```python
from build123d import *

# Parameters (mm, degrees)
SKETCH007_R      = 1.625
EXTRUDE007_DEPTH = 75
SKETCH006_R      = 1.625
EXTRUDE006_DEPTH = 10
EXTRUDE004_DEPTH = 20
SKETCH005_W      = 48
SKETCH005_H      = 25
SKETCH005_R      = 1.625
EXTRUDE005_DEPTH = 5
FILLET014_R      = 1
FILLET001_R      = 1
FILLET002_R      = 0.25


with BuildPart() as extrude007:
    # Sketch007 → Extrude007 (new body)
    with BuildSketch(Plane.YZ):
        with Locations((-8.1, 14.25)):
            Circle(SKETCH007_R)
    extrude(amount=EXTRUDE007_DEPTH)


with BuildPart() as cuts:
    # Sketch006 → Extrude006 (new body)
    with BuildSketch(Plane.XY):
        with Locations((29.75, -15.85)):
            Circle(SKETCH006_R)
    extrude(amount=-EXTRUDE006_DEPTH)

    # Fusion016: union Extrude007
    add(extrude007.part)


with BuildPart() as extrude004:
    # Sketch004 → Extrude004 (new body)
    with BuildSketch(Plane.XZ):
        Polygon((25, 0), (25, -4), (59.5, -4), (59.5, 21), (55.5, 21), (55.5, 0), align=None)
    extrude(amount=EXTRUDE004_DEPTH)


with BuildPart() as fillet002:
    # Sketch005 → Extrude005 (new body)
    with BuildSketch(Plane.XZ):
        with Locations((49, 8.5)):
            Rectangle(SKETCH005_W, SKETCH005_H)
        with Locations((67, 15)):
            Circle(SKETCH005_R, mode=Mode.SUBTRACT)
        with Locations((67, 2)):
            Circle(SKETCH005_R, mode=Mode.SUBTRACT)
    extrude(amount=EXTRUDE005_DEPTH)

    # Fusion015: union Extrude004
    add(extrude004.part)

    # Cut019: cut cuts
    add(cuts.part, mode=Mode.SUBTRACT)

    # Fillet014
    fillet014_edges = [fillet002.edges().sort_by_distance(p)[0] for p in [
        (57.5, -20, 21),
        (59.5, -20, 8.5),
        (55.5, -20, 10.5),
        (25, -20, -2),
        (42.25, -20, -4),
        (40.25, -20, 0),
    ]]
    fillet(fillet014_edges, radius=FILLET014_R)

    # Fillet001
    fillet001_edges = [fillet002.edges().sort_by_distance(p)[0] for p in [
        (66.25, -5, 21),
        (66.25, -5, -4),
        (73, -5, 8.5),
    ]]
    fillet(fillet001_edges, radius=FILLET001_R)

    # Fillet002
    fillet002_edges = [fillet002.edges().sort_by_distance(p)[0] for p in [
        (59.5, -9.725, 14.25),
        (28.125, -15.85, -4),
        (65.375, -5, 2),
        (65.375, -5, 15),
    ]]
    fillet(fillet002_edges, radius=FILLET002_R)


solid = fillet002.part
```
Can you work these out from the model? Positions are in its coordinate system, mm. A direction names the side the tool comes from. Coordinates: 2 decimals unless noted, no trailing zeros. Loops run counter-clockwise (first coordinate to the right, second up) from the corner with the lowest first, then second, coordinate; pieces in that order, holes last. Notation, with made-up numbers: (83, -36.5) - (130, -36.5) arc R16 cw to (130, -8.5) - close; hole circle Ø3 at (54.5, 67.5). An arc over 180 degrees is marked (long way). Answer as CSV lines item,"result". Start each with the question number.
1) Suppose I cut it at D-D (x = 29.75). Please give me the cut outline in (y, z) (3 decimals).
2) Suppose I cut it at C-C (y = -15.85). Please give me the cut outline in (x, z) (3 decimals).
3) Suppose I cut it at B-B (x = 67). Please give me the cut outline in (y, z) (3 decimals).
4) I need wall thicknesses on line 1 (Z direction, x = 67, y = -3.35) (3 decimals); line 2 (Z direction, x = 58.5, y = -8.1) (3 decimals); line 3 (Y direction, x = 57.55, z = 14.25) (3 decimals). Which ranges of each line are inside material? Lowest first, please. Write a range as from..to.
5) Suppose I cut it at A-A (z = 2). Please give me the cut outline in (x, y) (3 decimals).
6) For pin 1 (1 mm diameter, centred on x = 42, z = 13.5, fed in from +Y); pin 2 (4 mm diameter, centred on y = -8.1, z = 14.25, fed in from +X); pin 3 (10 mm diameter, centred on x = 65, z = 14, fed in from -Y); pin 4 (4 mm diameter, centred on x = 34.5, y = -13, fed in from +Z), each with a flat end and sliding along its axis, tell me the tip position at first contact or that it passes through.
7) Which directions (+Z, -Z, +X, -X, +Y, -Y) give clear straight access to the entire face, cutting with the end or side of a thin tool? Please do faces 4 (the flat face through (40, -5, 11)), 5 (the cylindrical face through (66.344, -4.699, -3.715)), 6 (the flat face through (66, -5, 9)).
8) Thinking about a two-plate mould opening in Y: for faces 1 (the cylindrical face through (68.5, -2.34, 14.38)), 2 (the cylindrical face through (28.127, -15.779, -1.849)), 3 (the cylindrical face through (59.199, -19.715, 8.675)), which applies, pulls with the +Y half, pulls with the -Y half, needs draft (parallel to the pull), parting line crosses it, or undercut?
Check result:
1,outline,"(-20, -3) arc R1 ccw to (-19, -4) - (-17.725, -4) arc R0.25 ccw to (-17.475, -3.75) - (-17.475, 0) - (-19, 0) arc R1 ccw to (-20, -1) - close; (-14.225, -3.75) arc R0.25 ccw to (-13.975, -4) - (0, -4) - (0, 21) - (-5, 21) - (-5, 0) - (-14.225, 0) - close"
2,outline,"(25, -4) - (27.875, -4) arc R0.25 ccw to (28.125, -3.75) - (28.125, 0) - (25, 0) - close; (31.375, -3.75) arc R0.25 ccw to (31.625, -4) - (59.5, -4) - (59.5, 21) - (55.5, 21) - (55.5, 0) - (31.375, 0) - close"
3,outline,"(-5, -3) arc R1 ccw to (-4, -4) - (0, -4) - (0, 0.375) - (-4.75, 0.375) arc R0.25 ccw to (-5, 0.125) - close; (-5, 3.875) arc R0.25 ccw to (-4.75, 3.625) - (0, 3.625) - (0, 13.375) - (-4.75, 13.375) arc R0.25 ccw to (-5, 13.125) - close; (-5, 16.875) arc R0.25 ccw to (-4.75, 16.625) - (0, 16.625) - (0, 21) - (-4, 21) arc R1 ccw to (-5, 20) - close"
4,line 1,"z = -4..0.375, 3.625..13.375, 16.625..21"
4,line 2,"z = -4..12.625, 15.875..21"
4,line 3,"y = -20..-9.725, -6.475..0"
5,outline,"(25, -5) - (55.5, -5) - (55.5, -19) arc R1 ccw to (56.5, -20) - (58.5, -20) arc R1 ccw to (59.5, -19) - (59.5, -5) - (65.125, -5) arc R0.25 ccw to (65.375, -4.75) - (65.375, 0) - (25, 0) - close; (68.625, -4.75) arc R0.25 ccw to (68.875, -5) - (72, -5) arc R1 ccw to (73, -4) - (73, 0) - (68.625, 0) - close"
6,pin 1,"stops at y = 0"
6,pin 2,"stops at x = 59.5"
6,pin 3,"stops at y = -5"
6,pin 4,"stops at z = 0"
7,face 4,"+Z, -X, -Y"
7,face 5,"-Z, +X, -Y"
7,face 6,"+Z, -Z, +X, -Y"
8,face 1,"needs draft"
8,face 2,"undercut"
8,face 3,"pulls with the -Y half"
